Verification items for this drawing (mm, ordinates from the low corner). A direction names the side the tool comes from. Round coordinates to 2 decimals unless told otherwise and drop trailing zeros. Order: outer loops, then holes, each group sorted by start corner. A loop starts at its lowest first (then second) coordinate and runs counter-clockwise, first axis right, second up. Notation, with made-up numbers: (-37, -22) - (12, -22) arc R24 cw to (12, -8) - close; hole circle Ø7 at (14.5, 50.5). An arc over 180 degrees is marked (long way). Use a Markdown table: item, result. Add a question column.
(1) Access from +Z, -Z, +X, -X, +Y, -Y to the whole of each face (thin tool, end or side, straight path). Record for the marked faces 4 and 5.
(2) Section check B-B on z = 8.25. Record the boundary of the cut face in (x, y), then the cut area to 3 significant figures.
(3) Mould release check, pull along Y, two halves, no side actions. Record for the marked faces 1, 2 and 3: released by +Y, released by -Y, zero draft, split by the parting line, or undercut.
(4) Thickness scan on line 1 along Y through (x, z) = (2.25, 7); line 2 along Z through (x, y) = (3.5, 2.75). Record the ranges inside material, lowest first. Write a range as [from, to].
(5) Gauge pin test, flat end, axial feed: P1, Ø1.7, axis at x = 3.5, y = 4.5, coming from the +Z side. Record the tip position at first contact, or that the pin passes through.
(6) Section check A-A on y = 5.5. Record the boundary of the cut face in (x, z), then the cut area to 3 significant figures.
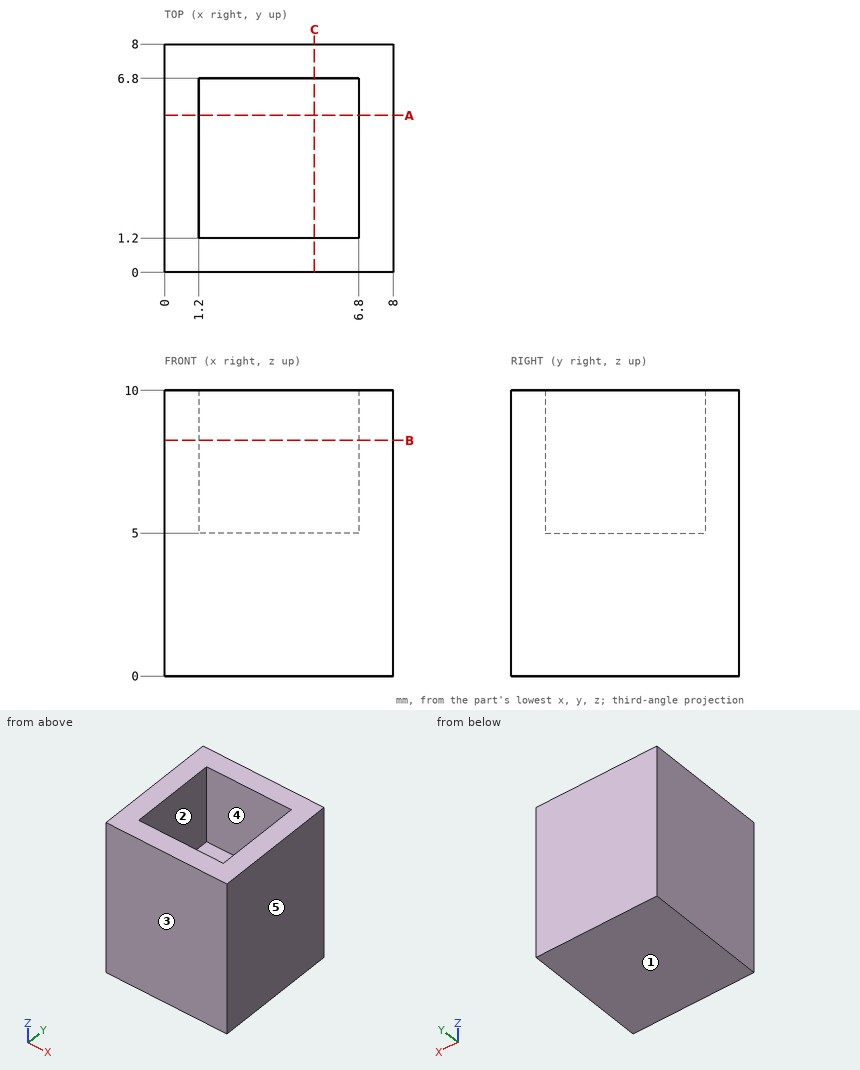
Check sheet entries:
| question | item | result |
|---|---|---|
| 1 | face 4 | +Z |
| 1 | face 5 | +Z, -Z, +X, +Y, -Y |
| 2 | outline | (0, 0) - (8, 0) - (8, 8) - (0, 8) - close; hole (1.2, 1.2) - (6.8, 1.2) - (6.8, 6.8) - (1.2, 6.8) - close |
| 2 | area | 32.6 mm2 |
| 3 | face 1 | zero draft |
| 3 | face 2 | undercut |
| 3 | face 3 | released by -Y |
| 4 | line 1 | y = [0, 1.2], [6.8, 8] |
| 4 | line 2 | z = [0, 5] |
| 5 | P1 | stops at z = 5 |
| 6 | outline | (0, 0) - (8, 0) - (8, 10) - (6.8, 10) - (6.8, 5) - (1.2, 5) - (1.2, 10) - (0, 10) - close |
| 6 | area | 52.0 mm2 |
